The figure shows three views and two pictorial views of one solid part (mm, origin at its lowest corner). Answer the questions. Coordinates: 2 decimals unless noted, no trailing zeros. Loops run counter-clockwise (first coordinate to the right, second up) from the corner with the lowest first, then second, coordinate; pieces in that order, holes last. Notation, with made-up numbers: M 10,-12 L 18,-12 A6 cw 18,-1 Z; hole C 56.25,42.5 d7. An arc over 180 degrees is marked long. Return JSON: item names as keys, results as strings. Group by question number.
1. Section B-B (x = 11.5) is taken. Write down the section's boundary in (y, z) (1 decimal).
2. Straight lines are drawn through the part: L1, parallel to Y at x = 19, z = 7.75 (1 decimal); L2, parallel to Y at x = 9.25, z = 8.5 (1 decimal); L3, parallel to X at y = 7.5, z = 10.5. For each, find the intervals that lie inside material, in ascending order. Write a range as from..to.
3. Section C-C (z = 5) is taken. Write down the section's boundary in (x, y) (1 decimal).
4. Given P1, Ø14.5, axis at x = 12.51, y = 13.59, coming from the -Z side, flat-ended and moving along its own axis, determine where the tip first touches the part or whether it passes through.
5. Section A-A (y = 16) is taken. Write down the section's boundary in (x, z) (1 decimal).
6. The mould has two halves that part along Y. Classify the marked faces 1, 2, 3 and 4: pulls with the +Y half, pulls with the -Y half, needs draft (parallel to the pull), parting line crosses it, or undercut.
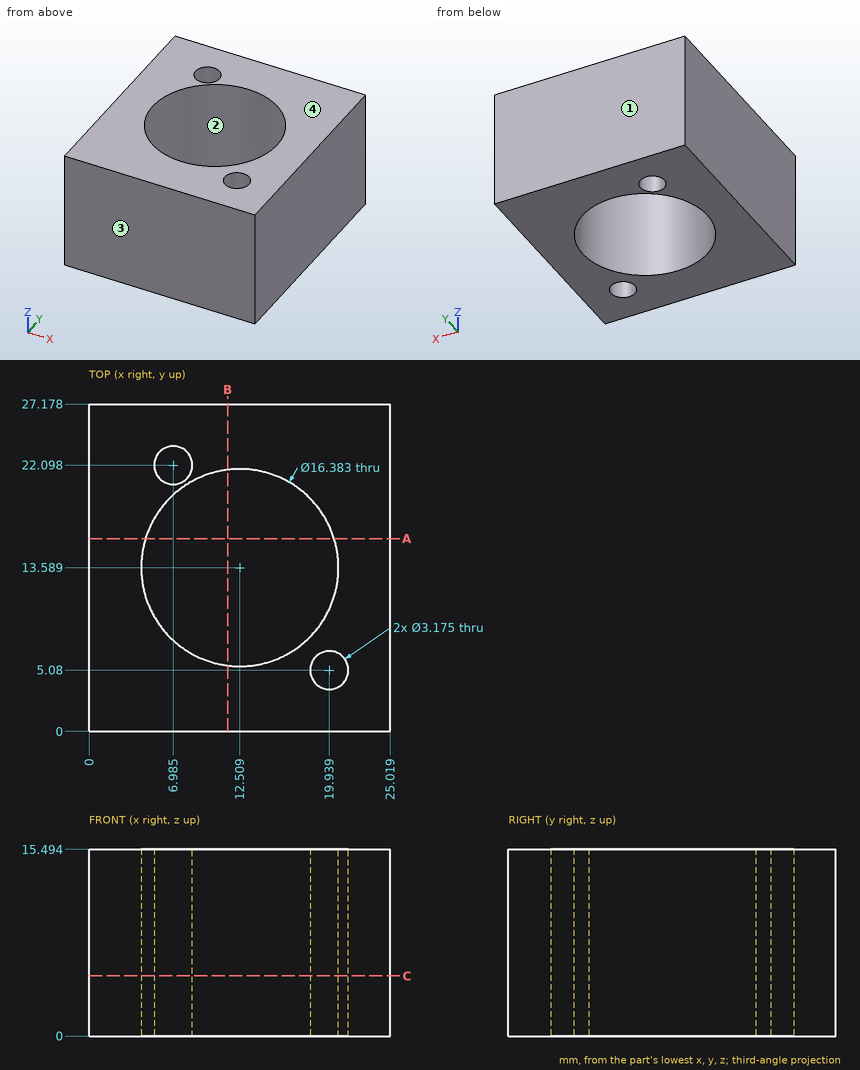
Worked out:
{
 "1": {"outline": "M 0,0 L 5.5,0 L 5.5,15.5 L 0,15.5 Z; M 21.7,0 L 27.2,0 L 27.2,15.5 L 21.7,15.5 Z"},
 "2": {"L1": "0..3.8, 6.4..8.6, 18.6..27.2", "L2": "0..6.1, 21.1..27.2", "L3": "0..7.03, 17.99..25.02"},
 "3": {"outline": "M 0,0 L 25,0 L 25,27.2 L 0,27.2 Z; hole C 12.5,13.6 d16.4; hole C 7,22.1 d3.2; hole C 19.9,5.1 d3.2"},
 "4": {"P1": "through"},
 "5": {"outline": "M 0,0 L 4.7,0 L 4.7,15.5 L 0,15.5 Z; M 20.3,0 L 25,0 L 25,15.5 L 20.3,15.5 Z"},
 "6": {"face 1": "pulls with the +Y half", "face 2": "undercut", "face 3": "pulls with the -Y half", "face 4": "needs draft"}
}
